```python
from build123d import *

# Parameters (mm, degrees)
SKETCH1_W           = 76
SKETCH1_H           = 28
SKETCH1_W_2         = 4.5
SKETCH1_H_2         = 2
BOSS_EXTRUDE1_DEPTH = 1
FILLET1_R           = 1


with BuildPart() as part:
    # Sketch1 → Boss-Extrude1 (new, symmetric)
    with BuildSketch(Plane.XY):
        Rectangle(SKETCH1_W, SKETCH1_H)
        with Locations((-32.5, -15)):
            Rectangle(SKETCH1_W_2, SKETCH1_H_2)
        with Locations((32.5, -15)):
            Rectangle(SKETCH1_W_2, SKETCH1_H_2)
        with Locations((0, 15)):
            Rectangle(SKETCH1_W_2, SKETCH1_H_2)
    extrude(amount=BOSS_EXTRUDE1_DEPTH, both=True)

    # Fillet1
    fillet1_edges = [part.edges().sort_by_distance(p)[0] for p in [
        (38, -14, 0),
        (34.75, -16, 0),
        (30.25, -16, 0),
        (-30.25, -16, 0),
        (-34.75, -16, 0),
        (-38, -14, 0),
        (-38, 14, 0),
        (38, 14, 0),
        (2.25, 16, 0),
        (-2.25, 16, 0),
    ]]
    fillet(fillet1_edges, radius=FILLET1_R)


solid = part.part
```
Verification items for the finished model (mm, model axes). A direction names the side the tool comes from. Give positions to 0.01 mm unless a question says otherwise; leave off trailing zeros. Order: outer loops, then holes, each group sorted by start corner. A loop starts at its lowest first (then second) coordinate and runs counter-clockwise, first axis right, second up. Notation, with made-up numbers: (-18, 79) -> (25, 79) arc R12 cw to (25, 101) -> close; hole circle Ø2 at (54.5, -8.75). An arc over 180 degrees is marked (long way). Use a Markdown table: item, result.
1) Section check A-A, the plane z = -0.7. Record the boundary of the cut face in (x, y).
Results:
| item | result |
|---|---|
| outline | (-38, -13) arc R1 ccw to (-37, -14) -> (-34.75, -14) -> (-34.75, -15) arc R1 ccw to (-33.75, -16) -> (-31.25, -16) arc R1 ccw to (-30.25, -15) -> (-30.25, -14) -> (30.25, -14) -> (30.25, -15) arc R1 ccw to (31.25, -16) -> (33.75, -16) arc R1 ccw to (34.75, -15) -> (34.75, -14) -> (37, -14) arc R1 ccw to (38, -13) -> (38, 13) arc R1 ccw to (37, 14) -> (2.25, 14) -> (2.25, 15) arc R1 ccw to (1.25, 16) -> (-1.25, 16) arc R1 ccw to (-2.25, 15) -> (-2.25, 14) -> (-37, 14) arc R1 ccw to (-38, 13) -> close |
2) Mould release check, pull along X, two halves, no side actions. Record for faces 6 (the flat face through (0, 16, 0)), 7 (the flat face through (0, -14, 0)), 8 (the flat face through (38, 0, 0)): pulls with the +X half, pulls with the -X half, needs draft (parallel to the pull), parting line crosses it, or undercut.
Results:
| item | result |
|---|---|
| face 6 | needs draft |
| face 7 | undercut |
| face 8 | pulls with the +X half |
3) Tool access check on faces 1 (the flat face through (36, -14, 0)), 2 (the flat face through (-20, 14, 0)), 3 (the flat face through (-36, -14, 0)), 4 (the flat face through (19, 14, 0)), 5 (the flat face through (-38, 0, 0)). Record the directions out of +Z, -Z, +X, -X, +Y, -Y that give a thin tool (end or side, any length) a straight path to the whole face; none if there is none.
Results:
| item | result |
|---|---|
| face 1 | +Z, -Z, +X, -Y |
| face 2 | +Z, -Z, -X, +Y |
| face 3 | +Z, -Z, -X, -Y |
| face 4 | +Z, -Z, +X, +Y |
| face 5 | +Z, -Z, -X, +Y, -Y |
4) Section check B-B, the plane x = -9. Record the boundary of the cut face in (y, z).
Results:
| item | result |
|---|---|
| outline | (-14, -1) -> (14, -1) -> (14, 1) -> (-14, 1) -> close |
5) Depth check by flat-ended pin: pin 1 Ø0.6 at (x, z) = (-36, 0) entering from -Y; pin 2 Ø1 at (x, z) = (20, -0.5) entering from +Y; pin 3 Ø0.5 at (y, z) = (14.5, -0.5) entering from -X. Enter the tip coordinate at first touch or a pass-through.
Results:
| item | result |
|---|---|
| pin 1 | y = -14 |
| pin 2 | y = 14 |
| pin 3 | x = -2.25 |
6) Material ranges on probe 1 along Y at (x, z) = (11, 0.8); probe 2 along Y at (x, z) = (0, 0.3), recorded low to high.
Results:
| item | result |
|---|---|
| probe 1 | -14 to 14 |
| probe 2 | -14 to 16 |
